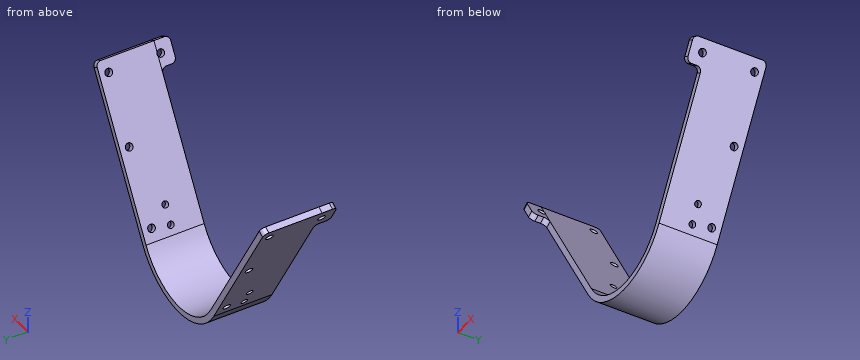
from build123d import *

# Parameters (mm, degrees)
BOSS_EXTRUDE10_DEPTH = 30.1625
SKETCH29_W           = 12.7
SKETCH29_H           = 7.9375
BOSS_EXTRUDE12_DEPTH = 6.35
CUT_EXTRUDE19_REACH  = 181.357
SKETCH30_R           = 1.651
CUT_EXTRUDE23_REACH  = 181.357
SKETCH38_R           = 1.905
FILLET24_R           = 2.54
CONVERT_SOLID1_DEPTH = 38.1


# Read off the part's stored shape, not the designer's step: Convert-Solid1
with BuildPart() as part:
    # Sketch28 → Boss-Extrude10 (new body)
    with BuildSketch(Plane(origin=(0, 38.1, 0), x_dir=(-1, 0, 0), z_dir=(0, -1, 0))):
        with BuildLine():
            Line((32.995567884, 114.3), (75.858067884, 40.059972261))
            Line((75.858067884, 40.059972261), (70.35880657, 36.884972261))
            Line((70.35880657, 36.884972261), (27.49630657, 111.125))
            ThreePointArc((27.49630657, 111.125), (0, 127), (-27.49630657, 111.125))
            Line((-27.49630657, 111.125), (-70.35880657, 36.884972261))
            Line((-70.35880657, 36.884972261), (-75.858067884, 40.059972261))
            Line((-75.858067884, 40.059972261), (-32.995567884, 114.3))
            ThreePointArc((-32.995567884, 114.3), (0, 133.35), (32.995567884, 114.3))
        make_face()
    extrude(amount=BOSS_EXTRUDE10_DEPTH)

    # Sketch29 → Boss-Extrude12 (add)
    with BuildSketch(Plane(origin=(-74.240027739, 0, -42.8625), x_dir=(-0.5, 0, 0.8660254037844387), z_dir=(-0.8660254037844387, 0, -0.5))):
        with Locations((-3.11391971, 3.96875)):
            Rectangle(SKETCH29_W, SKETCH29_H)
    boss_extrude12 = extrude(amount=-BOSS_EXTRUDE12_DEPTH)

    # Sketch30 → Cut-Extrude19 (cut, up to next)
    with BuildSketch(Plane(origin=(-74.240027739, 0, -42.8625), x_dir=(-0.5, 0, 0.8660254037844387), z_dir=(-0.8660254037844387, 0, -0.5)), mode=Mode.PRIVATE) as cut_extrude19_sk1:
        with Locations((-77.72641971, 23.8125)):
            Circle(SKETCH30_R)
    cut_extrude19_tool1 = extrude(cut_extrude19_sk1.sketch, amount=-CUT_EXTRUDE19_REACH, mode=Mode.PRIVATE) & part.part
    # Sketch30 → Cut-Extrude19 (cut, up to next)
    with BuildSketch(Plane(origin=(-74.240027739, 0, -42.8625), x_dir=(-0.5, 0, 0.8660254037844387), z_dir=(-0.8660254037844387, 0, -0.5)), mode=Mode.PRIVATE) as cut_extrude19_sk2:
        with Locations((-68.20141971, 23.8125)):
            Circle(SKETCH30_R)
    cut_extrude19_tool2 = extrude(cut_extrude19_sk2.sketch, amount=-CUT_EXTRUDE19_REACH, mode=Mode.PRIVATE) & part.part
    cut_extrude19_1 = cut_extrude19_tool1.solids().sort_by_distance((-35.376818, 23.8125, -110.175554))[0]
    add(cut_extrude19_1, mode=Mode.SUBTRACT)
    cut_extrude19_2 = cut_extrude19_tool2.solids().sort_by_distance((-40.139318, 23.8125, -101.926662))[0]
    add(cut_extrude19_2, mode=Mode.SUBTRACT)
    cut_extrude19 = cut_extrude19_1 + cut_extrude19_2  # Cut-Extrude19 as one shape, for the pattern or mirror that repeats it

    # Sketch38 → Cut-Extrude23 (cut, up to next)
    with BuildSketch(Plane(origin=(-74.240027739, 0, -42.8625), x_dir=(-0.5, 0, 0.8660254037844387), z_dir=(-0.8660254037844387, 0, -0.5)), mode=Mode.PRIVATE) as cut_extrude23_sk1:
        with Locations((-76.13891971, 33.3375)):
            Circle(SKETCH38_R)
    cut_extrude23_tool1 = extrude(cut_extrude23_sk1.sketch, amount=-CUT_EXTRUDE23_REACH, mode=Mode.PRIVATE) & part.part
    # Sketch38 → Cut-Extrude23 (cut, up to next)
    with BuildSketch(Plane(origin=(-74.240027739, 0, -42.8625), x_dir=(-0.5, 0, 0.8660254037844387), z_dir=(-0.8660254037844387, 0, -0.5)), mode=Mode.PRIVATE) as cut_extrude23_sk2:
        with Locations((-38.03891971, 33.3375)):
            Circle(SKETCH38_R)
    cut_extrude23_tool2 = extrude(cut_extrude23_sk2.sketch, amount=-CUT_EXTRUDE23_REACH, mode=Mode.PRIVATE) & part.part
    # Sketch38 → Cut-Extrude23 (cut, up to next)
    with BuildSketch(Plane(origin=(-74.240027739, 0, -42.8625), x_dir=(-0.5, 0, 0.8660254037844387), z_dir=(-0.8660254037844387, 0, -0.5)), mode=Mode.PRIVATE) as cut_extrude23_sk3:
        with Locations((-3.11391971, 33.3375)):
            Circle(SKETCH38_R)
    cut_extrude23_tool3 = extrude(cut_extrude23_sk3.sketch, amount=-CUT_EXTRUDE23_REACH, mode=Mode.PRIVATE) & part.part
    # Sketch38 → Cut-Extrude23 (cut, up to next)
    with BuildSketch(Plane(origin=(-74.240027739, 0, -42.8625), x_dir=(-0.5, 0, 0.8660254037844387), z_dir=(-0.8660254037844387, 0, -0.5)), mode=Mode.PRIVATE) as cut_extrude23_sk4:
        with Locations((-3.11391971, 6.35)):
            Circle(SKETCH38_R)
    cut_extrude23_tool4 = extrude(cut_extrude23_sk4.sketch, amount=-CUT_EXTRUDE23_REACH, mode=Mode.PRIVATE) & part.part
    cut_extrude23_1 = cut_extrude23_tool1.solids().sort_by_distance((-36.170568, 33.3375, -108.800739))[0]
    add(cut_extrude23_1, mode=Mode.SUBTRACT)
    cut_extrude23_2 = cut_extrude23_tool2.solids().sort_by_distance((-55.220568, 33.3375, -75.805171))[0]
    add(cut_extrude23_2, mode=Mode.SUBTRACT)
    cut_extrude23_3 = cut_extrude23_tool3.solids().sort_by_distance((-72.683068, 33.3375, -45.559234))[0]
    add(cut_extrude23_3, mode=Mode.SUBTRACT)
    cut_extrude23_4 = cut_extrude23_tool4.solids().sort_by_distance((-72.683068, 6.35, -45.559234))[0]
    add(cut_extrude23_4, mode=Mode.SUBTRACT)
    cut_extrude23 = cut_extrude23_1 + cut_extrude23_2 + cut_extrude23_3 + cut_extrude23_4  # Cut-Extrude23 as one shape, for the pattern or mirror that repeats it

    # Mirror7: Boss-Extrude12, Cut-Extrude19, Cut-Extrude23 across plane
    add(boss_extrude12.mirror(Plane(origin=(0, 0, 0), x_dir=(0, 0, 1), z_dir=(1, 0, 0))))
    add(cut_extrude19.mirror(Plane(origin=(0, 0, 0), x_dir=(0, 0, 1), z_dir=(1, 0, 0))), mode=Mode.SUBTRACT)
    add(cut_extrude23.mirror(Plane(origin=(0, 0, 0), x_dir=(0, 0, 1), z_dir=(1, 0, 0))), mode=Mode.SUBTRACT)

    # Fillet24
    fillet24_edges = [part.edges().sort_by_distance(p)[0] for p in [
        (73.108437227, 38.1, -38.472472261),
        (-73.108437227, 0, -38.472472261),
        (-66.758437227, 0, -49.470994889),
        (-66.758437227, 7.9375, -49.470994889),
        (73.108437227, 0, -38.472472261),
        (66.758437227, 7.9375, -49.470994889),
        (66.758437227, 0, -49.470994889),
        (-73.108437227, 38.1, -38.472472261),
    ]]
    fillet(fillet24_edges, radius=FILLET24_R)

    # Convert-Solid1 outline → Convert-Solid1 (cut)
    with BuildSketch(Plane(origin=(0, 0, 0), x_dir=(1, 0, 0), z_dir=(0, 1, 0))):
        with BuildLine():
            ThreePointArc((-30.245937227, 112.7125), (0, 130.175), (30.245937227, 112.7125))
            Line((30.245937227, 112.7125), (73.108437227, 38.472472261))
            Line((73.108437227, 38.472472261), (75.858067884, 40.059972261))
            Line((75.858067884, 40.059972261), (32.995567884, 114.3))
            ThreePointArc((32.995567884, 114.3), (0, 133.35), (-32.995567884, 114.3))
            Line((-32.995567884, 114.3), (-75.858067884, 40.059972261))
            Line((-75.858067884, 40.059972261), (-73.108437227, 38.472472261))
            Line((-73.108437227, 38.472472261), (-30.245937227, 112.7125))
        make_face()
    extrude(amount=CONVERT_SOLID1_DEPTH, mode=Mode.SUBTRACT)


solid = part.part
Geometry check sheet. Reference: the model listing, model coordinates, mm. Give positions to 0.01 mm unless a question says otherwise; leave off trailing zeros. Write each loop counter-clockwise with the first axis right and the second up, starting at its lowest first coordinate (ties: lowest second). Pieces come first, ordered by that corner, then holes. Notation, with made-up numbers: M 77,29 L 127,29 A23 cw 127,55 Z; hole C -10.5,14.5 d4. An arc over 180 degrees is marked long. Answer as CSV lines item,"result". Start each with the question number.
Q1. Section check A-A, the plane z = -54. Record the cut outline in (x, y), then the cut area to 3 significant figures.
Q2. Go/stop test with flat-tipped pins: pin 1 (8 mm diameter, centred on x = 57.5, z = -67.5, fed in from -Y); pin 2 (3 mm diameter, centred on y = 12.5, z = -46.5, fed in from -X); pin 3 (1.5 mm diameter, centred on x = 33.5, y = 9, fed in from -Z). Record where each tip stops, or that it passes through.
Q3. Material ranges on L1, parallel to X at y = 28, z = -91; L2, parallel to X at y = 35, z = -68.5; L3, parallel to Z at x = 5.5, y = 18, recorded low to high.
Q4. Section check D-D, the plane x = 44. Record the cut outline in (y, z), then the cut area to 3 significant figures.
Q5. Section check C-C, the plane z = -119. Record the cut outline in (x, y), then the cut area to 3 significant figures.
Geometry says:
1,outline,"M -64.14,7.94 L -60.48,7.94 L -60.48,38.1 L -64.14,38.1 Z; M 60.48,7.94 L 64.14,7.94 L 64.14,38.1 L 60.48,38.1 Z"
1,area,"221 mm^2"
2,pin 1,"y = 7.94"
2,pin 2,"x = -69.34"
2,pin 3,"z = -108.38"
3,L1,"-42.78 to -39.12, 39.12 to 42.78"
3,L2,"-55.77 to -52.11, 52.11 to 55.77"
3,L3,"-129.74 to -126.52"
4,outline,"M 7.94,-88.89 L 38.1,-88.89 L 38.1,-82.54 L 7.94,-82.54 Z"
4,area,"192 mm^2"
5,outline,"M -25.61,7.94 L -21.07,7.94 L -21.07,38.1 L -25.61,38.1 Z; M 21.07,7.94 L 25.61,7.94 L 25.61,38.1 L 21.07,38.1 Z"
5,area,"274 mm^2"
